Work out the finished part from the listing and answer in its coordinate system (mm). A direction names the side the tool comes from. Coordinates: 2 decimals unless noted, no trailing zeros. Loops run counter-clockwise (first coordinate to the right, second up) from the corner with the lowest first, then second, coordinate; pieces in that order, holes last. Notation, with made-up numbers: (9.5, 80) - (29.5, 80) arc R18 cw to (29.5, 93) - close; hole circle Ø6 at (48.5, 31.5). An arc over 180 degrees is marked (long way). Write each question's results on one line, items separated by ' | '. Start each with the question number.
1. A cutting plane is placed at A-A on z = 0. Determine the outline of the cut face in (x, y).
2. Which of the six approach directions +Z, -Z, +X, -X, +Y, -Y give full straight-line access (tool end or side, diameter ignored) to faces 1 (the cylindrical face through (-2.515, 19.737, -1.928)), 2 (the flat face through (0, 0, 0))?
3. Find the intervals of material crossed by line 1 along Y through (x, z) = (-4.75, 3.75); line 2 along Z through (x, y) = (6.25, 6.25); line 3 along X through (y, z) = (8.5, 7.5), in increasing order. Write a range as [from, to].
4. A cutting plane is placed at B-B on x = 0. Determine the outline of the cut face in (y, z).
5. A cutting plane is placed at C-C on y = 3. Determine the outline of the cut face in (x, z), then the cut area to 3 significant figures.
6. A cutting plane is placed at D-D on y = 11.25. Determine the outline of the cut face in (x, z).
7. Each of these flat-tipped pins is pushed along its axis until it touches: P1, Ø8, axis at x = -8, y = 21, coming from the +Z side; P2, Ø8, axis at x = -6, y = 17.5, coming from the +Z side; P3, Ø6, axis at x = 4.5, y = 11.5, coming from the +Z side; P4, Ø1, axis at x = -0.5, y = 22.5, coming from the +Z side. Where does it stop, or does it pass through?
from build123d import *

# Parameters (mm, degrees)
CHAMFER1_SIZE = 1.524


with BuildPart() as part:
    # Sketch1 → Revolve1 (revolve)
    with BuildSketch(Plane.XY):
        with BuildLine():
            Line((0, 0), (0, 26.9748))
            Line((0, 26.9748), (3.16865, 26.9748))
            Line((3.16865, 26.9748), (3.16865, 12.7))
            Line((3.16865, 12.7), (7.9375, 12.7))
            ThreePointArc((7.9375, 12.7), (8.777939273, 9.148340087), (11.120996905, 6.35))
            Line((11.120996905, 6.35), (11.120996905, 0))
            Line((11.120996905, 0), (0, 0))
        make_face()
    revolve(axis=Axis((0, 0, 0), (0, -1, 0)))

    # Chamfer1
    chamfer1_edges = [part.edges().sort_by_distance(p)[0] for p in [
        (-11.120996905, 0, 0),
    ]]
    chamfer(chamfer1_edges, length=CHAMFER1_SIZE)


solid = part.part
Values:
1) outline: (-11.12, 1.52) - (-9.6, 0) - (9.6, 0) - (11.12, 1.52) - (11.12, 6.35) arc R7.92 cw to (7.94, 12.7) - (3.17, 12.7) - (3.17, 26.97) - (-3.17, 26.97) - (-3.17, 12.7) - (-7.94, 12.7) arc R7.92 cw to (-11.12, 6.35) - close
2) face 1: +Y | face 2: +Z, -Z, +X, -X, -Y
3) line 1: [0, 12.7] | line 2: [-9.2, 9.2] | line 3: [-5.23, 5.23]
4) outline: (0, -9.6) - (1.52, -11.12) - (6.35, -11.12) arc R7.92 cw to (12.7, -7.94) - (12.7, -3.17) - (26.97, -3.17) - (26.97, 3.17) - (12.7, 3.17) - (12.7, 7.94) arc R7.92 cw to (6.35, 11.12) - (1.52, 11.12) - (0, 9.6) - close
5) outline: circle Ø22.24 at (0, 0) | area: 389 mm^2
6) outline: circle Ø16.14 at (0, 0)
7) P1: through | P2: z = 2.46 | P3: z = 8.39 | P4: z = 3.17
